Part model, mm, in its own coordinate system. Face numbers are marked on the shaded views. Coordinates: 2 decimals unless noted, no trailing zeros. Order: outer loops, then holes, each group sorted by start corner. A loop starts at its lowest first (then second) coordinate and runs counter-clockwise, first axis right, second up. Notation, with made-up numbers: M -39,82 L -3,82 A5 cw -3,91 Z; hole C 24,-13.5 d3. An arc over 180 degrees is marked long. Answer in a Markdown table with one row per item. Add a question column.
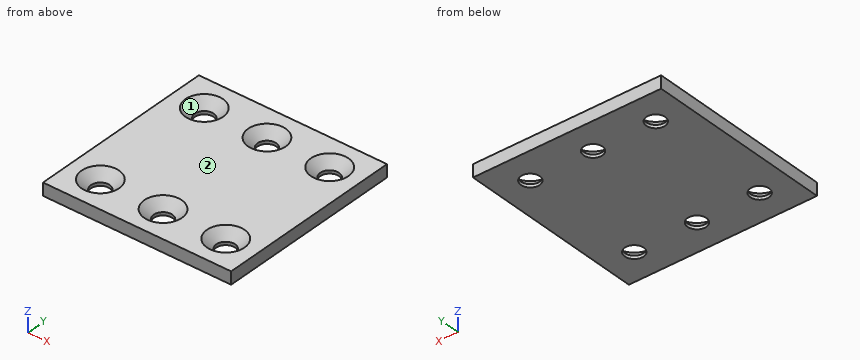
from build123d import *

# Parameters (mm, degrees)
SKETCH1_W           = 60
SKETCH1_H           = 60
BOSS_EXTRUDE1_DEPTH = 2
SKETCH2_R           = 3
CUT_EXTRUDE1_DEPTH  = 5
CHAMFER1_SIZE       = 3


with BuildPart() as part:
    # Sketch1 → Boss-Extrude1 (new body, symmetric)
    with BuildSketch(Plane.XY):
        Rectangle(SKETCH1_W, SKETCH1_H)
    extrude(amount=BOSS_EXTRUDE1_DEPTH, both=True)

    # Sketch2 → Cut-Extrude1 (cut, through all)
    with BuildSketch(Plane.XY.offset(2)):
        with Locations((0, 20)):
            Circle(SKETCH2_R)
        with Locations((0, -20)):
            Circle(SKETCH2_R)
        with Locations((20, -20)):
            Circle(SKETCH2_R)
        with Locations((-20, -20)):
            Circle(SKETCH2_R)
        with Locations((-20, 20)):
            Circle(SKETCH2_R)
        with Locations((20, 20)):
            Circle(SKETCH2_R)
    extrude(amount=-CUT_EXTRUDE1_DEPTH, mode=Mode.SUBTRACT)

    # Chamfer1
    chamfer1_edges = [part.edges().sort_by_distance(p)[0] for p in [
        (-3, -20, 2),
        (17, -20, 2),
        (-23, -20, 2),
        (-23, 20, 2),
        (17, 20, 2),
        (-3, 20, 2),
    ]]
    chamfer(chamfer1_edges, length=CHAMFER1_SIZE)


solid = part.part
(1) Slice it at A-A (y = -20). List the corners of the cut face in (x, z), and give its area (3 significant figures).
(2) Slice it at D-D (x = -19.5). State how many separate pieces and enclosed holes the cut face has, and give its area (3 significant figures).
(3) Wall check: line 1 (Y direction, x = -20, z = -1.65); line 2 (X direction, y = -19, z = -0.85); line 3 (Y direction, x = -20.5, z = 0.8). Give the ranges that are in metal, low to high.
(4) Pull direction Y, two halves, no side cores. Call the marked faces 1 and 2: pulls with the +Y half, pulls with the -Y half, needs draft (parallel to the pull), parting line crosses it, or undercut.
(5) Slice it at C-C (x = 20). List the corners of the cut face in (y, z), and give its area (3 significant figures).
(6) Drop a flat-ended pin along its axis: P1, Ø5.5, axis at x = 20, y = -20, coming from the +Z side. Give the stop position or say it passes through.
(7) Slice it at B-B (z = -0.25). List the corners of the cut face in (x, y), and give its area (3 significant figures).
Computed:
| question | item | result |
|---|---|---|
| 1 | outline | M -30,-2 L -23,-2 L -23,-1 L -26,2 L -30,2 Z; M -17,-2 L -3,-2 L -3,-1 L -6,2 L -14,2 L -17,-1 Z; M 3,-2 L 17,-2 L 17,-1 L 14,2 L 6,2 L 3,-1 Z; M 23,-2 L 30,-2 L 30,2 L 26,2 L 23,-1 Z |
| 1 | area | 141 mm^2 |
| 2 | separate pieces | 3 |
| 2 | enclosed holes | 0 |
| 2 | area | 175 mm^2 |
| 3 | line 1 | y = -30 to -23, -17 to 17, 23 to 30 |
| 3 | line 2 | x = -30 to -22.99, -17.01 to -2.99, 2.99 to 17.01, 22.99 to 30 |
| 3 | line 3 | y = -30 to -24.77, -15.23 to 15.23, 24.77 to 30 |
| 4 | face 1 | undercut |
| 4 | face 2 | needs draft |
| 5 | outline | M -30,-2 L -23,-2 L -23,-1 L -26,2 L -30,2 Z; M -17,-2 L 17,-2 L 17,-1 L 14,2 L -14,2 L -17,-1 Z; M 23,-2 L 30,-2 L 30,2 L 26,2 L 23,-1 Z |
| 5 | area | 174 mm^2 |
| 6 | P1 | passes through |
| 7 | outline | M -30,-30 L 30,-30 L 30,30 L -30,30 Z; hole C -20,-20 d7.5; hole C -20,20 d7.5; hole C 0,-20 d7.5; hole C 0,20 d7.5; hole C 20,-20 d7.5; hole C 20,20 d7.5 |
| 7 | area | 3,330 mm^2 |
